Can you work these out from the drawing? Everything is in mm from the part's minimum corner. Coordinates: 2 decimals unless noted, no trailing zeros. Loops run counter-clockwise (first coordinate to the right, second up) from the corner with the lowest first, then second, coordinate; pieces in that order, holes last. Notation, with made-up numbers: M -1.5,46 L 34.5,46 A14 ccw 34.5,53 Z; hole C 49,32.25 d7. An arc over 180 degrees is marked long. Use CSV: the item, a comma, the result in double quotes. Start each with the question number.
Q1. If we section it at B-B (z = 30): Please give me the cut outline in (x, y).
Q2. If we section it at A-A (x = 799.5): Please give me the cut outline in (y, z).
Q3. Please list where this line runs through material, in increasing order: probe 1 along Z at (x, y) = (624, 14). Write a range as [from, to].
Q4. For pin 1 Ø8 at (x, z) = (364.5, 8.5) entering from -Y, with a flat end and sliding along its axis, tell me the tip position at first contact or that it passes through.
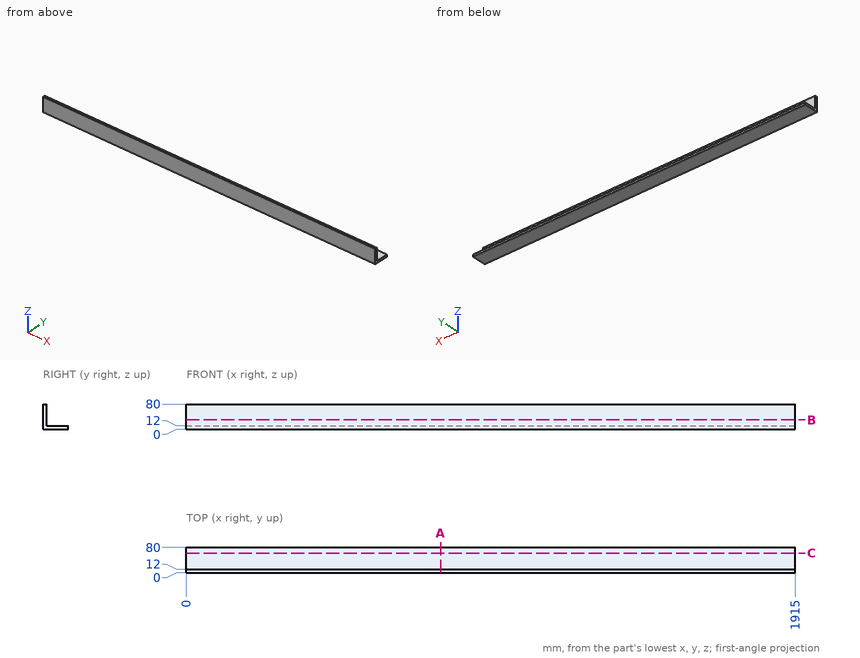
Results below:
1,outline,"M 0,0 L 1915,0 L 1915,12 L 0,12 Z"
2,outline,"M 0,0 L 80,0 L 80,12 L 12,12 L 12,80 L 0,80 Z"
3,probe 1,"[0, 12]"
4,pin 1,"y = 0"
